from build123d import *

# Parameters (mm, degrees)
SKETCH1_W               = 74
SKETCH1_H               = 51
BOSS_EXTRUDE1_DEPTH     = 1.6
SKETCH2_W               = 31
SKETCH2_H               = 36
BOSS_EXTRUDE2_DEPTH     = 5
SKETCH3_W               = 14
SKETCH3_H               = 15
BOSS_EXTRUDE3_DEPTH     = 8
SKETCH4_W               = 6
SKETCH4_H               = 49
BOSS_EXTRUDE4_DEPTH     = 4.5
CUT_EXTRUDE1_DEPTH      = 8.5
CUT_EXTRUDE1_DEPTH_BACK = 91.227490268
SKETCH6_R               = 1.5


with BuildPart() as part:
    # Sketch1 → Boss-Extrude1 (new body)
    with BuildSketch(Plane.XY):
        with Locations((37, 25.5)):
            Rectangle(SKETCH1_W, SKETCH1_H)
    extrude(amount=BOSS_EXTRUDE1_DEPTH)

    # Sketch2 → Boss-Extrude2 (add)
    with BuildSketch(Plane.XY.offset(1.6)):
        with Locations((41.5, 24)):
            Rectangle(SKETCH2_W, SKETCH2_H)
    extrude(amount=BOSS_EXTRUDE2_DEPTH)

    # Sketch3 → Boss-Extrude3 (add)
    with BuildSketch(Plane.XY.offset(1.6)):
        with Locations((6, 9.86)):
            Rectangle(SKETCH3_W, SKETCH3_H)
    extrude(amount=BOSS_EXTRUDE3_DEPTH)

    # Sketch4 → Boss-Extrude4 (add)
    with BuildSketch(Plane(origin=(0, 0, 0), x_dir=(-1, 0, 0), z_dir=(0, 0, -1))):
        with Locations((-63, 25.5)):
            Rectangle(SKETCH4_W, SKETCH4_H)
    extrude(amount=BOSS_EXTRUDE4_DEPTH)

    # Sketch6 → Cut-Extrude1 (cut, two sides: drawn at the far end of the back side and taken through both)
    with BuildSketch(Plane.XY.offset(1.6).offset(-CUT_EXTRUDE1_DEPTH_BACK)):
        with Locations(Location((55, 32, 0), (0, 0, 180))):
            Circle(SKETCH6_R)
        with Locations(Location((24, 25.5, 0), (0, 0, 180))):
            Circle(SKETCH6_R)
    extrude(amount=CUT_EXTRUDE1_DEPTH + CUT_EXTRUDE1_DEPTH_BACK, mode=Mode.SUBTRACT)


solid = part.part
Verification items for the finished model (mm, model axes). A direction names the side the tool comes from. Give positions to 0.01 mm unless a question says otherwise; leave off trailing zeros. Order: outer loops, then holes, each group sorted by start corner. A loop starts at its lowest first (then second) coordinate and runs counter-clockwise, first axis right, second up. Notation, with made-up numbers: (31.25, 31.5) -> (56.25, 31.5) arc R25 cw to (56.25, 70.5) -> close; hole circle Ø7 at (33.5, 37.5). An arc over 180 degrees is marked (long way). Answer as CSV lines item,"result".
Q1. Sectioned sample at C-C on x = 55. Record the cut outline in (y, z), plus the area to 3 significant figures.
Solutions:
outline,"(0, 0) -> (30.5, 0) -> (30.5, 6.6) -> (6, 6.6) -> (6, 1.6) -> (0, 1.6) -> close; (33.5, 0) -> (51, 0) -> (51, 1.6) -> (42, 1.6) -> (42, 6.6) -> (33.5, 6.6) -> close"
area,"242 mm²"
Q2. Scan lines: probe 1 along Y at (x, z) = (24, 0.8); probe 2 along Y at (x, z) = (55, 2.25); probe 3 along X at (y, z) = (18.5, 5.5). Record each from-to range of solid material in increasing order.
Solutions:
probe 1,"y = 0 to 24, 27 to 51"
probe 2,"y = 6 to 30.5, 33.5 to 42"
probe 3,"x = 26 to 57"
Q3. Sectioned sample at B-B on y = 32. Record the cut outline in (x, z), plus the area to 3 significant figures.
Solutions:
outline,"(0, 0) -> (53.5, 0) -> (53.5, 6.6) -> (26, 6.6) -> (26, 1.6) -> (0, 1.6) -> close; (56.5, 0) -> (60, 0) -> (60, -4.5) -> (66, -4.5) -> (66, 0) -> (74, 0) -> (74, 1.6) -> (57, 1.6) -> (57, 6.6) -> (56.5, 6.6) -> close"
area,"281 mm²"
Q4. Access from +Z, -Z, +X, -X, +Y, -Y to the whole of each face (thin tool, end or side, straight path). Record for faces 5 (the flat face through (57, 24, 4)), 6 (the flat face through (13, 10, 6)), 7 (the flat face through (66, 25, -2)), 8 (the flat face through (0, 25, 1)).
Solutions:
face 5,"+Z, +X, +Y, -Y"
face 6,"+Z, +Y, -Y"
face 7,"-Z, +X, +Y, -Y"
face 8,"-Z, -X, +Y, -Y"
Q5. Sectioned sample at D-D on y = 14.5. Record the cut outline in (x, z).
Solutions:
outline,"(-1, 1.6) -> (0, 1.6) -> (0, 0) -> (60, 0) -> (60, -4.5) -> (66, -4.5) -> (66, 0) -> (74, 0) -> (74, 1.6) -> (57, 1.6) -> (57, 6.6) -> (26, 6.6) -> (26, 1.6) -> (13, 1.6) -> (13, 9.6) -> (-1, 9.6) -> close"
Q6. Sectioned sample at A-A on z = 4.5. Record the cut outline in (x, y), plus the area to 3 significant figures.
Solutions:
outline,"(-1, 2.36) -> (13, 2.36) -> (13, 17.36) -> (-1, 17.36) -> close; (26, 6) -> (57, 6) -> (57, 42) -> (26, 42) -> close; hole circle Ø3 at (55, 32)"
area,"1,320 mm²"
Q7. Depth check by flat-ended pin: pin 1 (0.8 mm diameter, centred on y = 24, z = 0.5, fed in from -X); pin 2 (6.5 mm diameter, centred on y = 13, z = 6.5, fed in from +X); pin 3 (1 mm diameter, centred on x = 37.5, z = 4.5, fed in from -Y). Enter the tip coordinate at first touch or a pass-through.
Solutions:
pin 1,"stops at x = 0"
pin 2,"stops at x = 57"
pin 3,"stops at y = 6"
Q8. Release check for a two-part mould opening along Y. For faces 1 (the flat face through (41, 42, 4)), 2 (the cylindrical face through (24, 24, 1)), 3 (the flat face through (-1, 10, 6)), 4 (the cylindrical face through (53.57, 31.55, 3.25)) record: +Y half, -Y half, draft (parallel to the pull), parting line (faces both ways), or undercut.
Solutions:
face 1,"+Y half"
face 2,"undercut"
face 3,"draft"
face 4,"undercut"
